```python
from build123d import *

# Parameters (mm, degrees)
P_IDAT_VYSUNUT_M1_DEPTH = 6
M6_D_RA_S_V_L_1_D       = 6.6
SKICA5_W                = 8
SKICA5_H                = 8
P_IDAT_VYSUNUT_M2_DEPTH = 2


with BuildPart() as part:
    # Skica1 → Přidat vysunutím1 (new body)
    with BuildSketch(Plane.XY):
        with BuildLine():
            Line((0, 0), (57, 0))
            ThreePointArc((57, 0), (59.121320344, 0.878679656), (60, 3))
            Line((60, 3), (60, 27))
            ThreePointArc((60, 27), (59.121320344, 29.121320344), (57, 30))
            Line((57, 30), (33, 30))
            ThreePointArc((33, 30), (30.878679656, 30.878679656), (30, 33))
            Line((30, 33), (30, 57))
            ThreePointArc((30, 57), (29.121320344, 59.121320344), (27, 60))
            Line((27, 60), (3, 60))
            ThreePointArc((3, 60), (0.878679656, 59.121320344), (0, 57))
            Line((0, 57), (0, 0))
        make_face()
    extrude(amount=P_IDAT_VYSUNUT_M1_DEPTH)

    # M6 díra s vůlí1 (through all)
    with Locations(Plane.XY.offset(6)):
        with Locations((45, 15), (15, 45)):
            Hole(M6_D_RA_S_V_L_1_D / 2)

    # Skica5 → Přidat vysunutím2 (add)
    with BuildSketch(Plane.XY.offset(6)):
        with BuildLine():
            ThreePointArc((19, 41.225082782), (15, 39.5), (11, 41.225082782))
            Line((11, 41.225082782), (11, 32.5))
            Line((11, 32.5), (19, 32.5))
            Line((19, 32.5), (19, 41.225082782))
        make_face()
        with BuildLine():
            Line((19, 57.5), (11, 57.5))
            Line((11, 57.5), (11, 48.774917218))
            ThreePointArc((11, 48.774917218), (15, 50.5), (19, 48.774917218))
            Line((19, 48.774917218), (19, 57.5))
        make_face()
        with BuildLine():
            Line((41.225082782, 19), (32.5, 19))
            Line((32.5, 19), (32.5, 11))
            Line((32.5, 11), (41.225082782, 11))
            ThreePointArc((41.225082782, 11), (39.5, 15), (41.225082782, 19))
        make_face()
        with BuildLine():
            Line((57.5, 19), (48.774917218, 19))
            ThreePointArc((48.774917218, 19), (50.050348735, 17.178067412), (50.5, 15))
            ThreePointArc((50.5, 15), (50.050348735, 12.821932588), (48.774917218, 11))
            Line((48.774917218, 11), (57.5, 11))
            Line((57.5, 11), (57.5, 19))
        make_face()
        with Locations((15, 15)):
            Rectangle(SKICA5_W, SKICA5_H)
    extrude(amount=P_IDAT_VYSUNUT_M2_DEPTH)


solid = part.part
```
The model under review builds one solid part; all positions refer to its coordinate system, in mm. A direction names the side the tool comes from. Round coordinates to 2 decimals unless told otherwise and drop trailing zeros. Write each loop counter-clockwise with the first axis right and the second up, starting at its lowest first coordinate (ties: lowest second). Pieces come first, ordered by that corner, then holes. Notation, with made-up numbers: (52, 78) -> (89, 78) arc R15 cw to (89, 90) -> close; hole circle Ø6 at (13.5, 78.25). An arc over 180 degrees is marked (long way). Use CSV: the item, a comma, the result in double quotes.
Q1. Consider section D-D (z = 3). Give the boundary of the cut face in (x, y).
Checks:
outline,"(0, 0) -> (57, 0) arc R3 ccw to (60, 3) -> (60, 27) arc R3 ccw to (57, 30) -> (33, 30) arc R3 cw to (30, 33) -> (30, 57) arc R3 ccw to (27, 60) -> (3, 60) arc R3 ccw to (0, 57) -> close; hole circle Ø6.6 at (15, 45); hole circle Ø6.6 at (45, 15)"
Q2. Consider section A-A (y = 45). Give the boundary of the cut face in (x, z), then the cut area to 3 significant figures.
Checks:
outline,"(0, 0) -> (11.7, 0) -> (11.7, 6) -> (0, 6) -> close; (18.3, 0) -> (30, 0) -> (30, 6) -> (18.3, 6) -> close"
area,"140 mm²"
Q3. For pin 1 Ø5 at (x, y) = (6, 6) entering from +Z; pin 2 Ø1 at (y, z) = (52, 7) entering from +X; pin 3 Ø1.8 at (x, z) = (41, 4) entering from +Y, all flat-tipped, find the tip position at first contact; note any pin that passes through.
Checks:
pin 1,"z = 6"
pin 2,"x = 19"
pin 3,"y = 30"
Q4. Consider section B-B (z = 6.75). Give the boundary of the cut face in (x, y), then the cut area to 3 significant figures.
Checks:
outline,"(11, 11) -> (19, 11) -> (19, 19) -> (11, 19) -> close; (11, 32.5) -> (19, 32.5) -> (19, 41.23) arc R5.5 cw to (11, 41.23) -> close; (11, 48.77) arc R5.5 cw to (19, 48.77) -> (19, 57.5) -> (11, 57.5) -> close; (32.5, 11) -> (41.23, 11) arc R5.5 cw to (41.23, 19) -> (32.5, 19) -> close; (48.77, 11) -> (57.5, 11) -> (57.5, 19) -> (48.77, 19) arc R5.5 cw to start"
area,"305 mm²"
Q5. Mouldability with a two-part tool opening along X and no side actions: class faces 1 (the cylindrical face through (59.14, 29.1, 2.96)), 2 (the flat face through (19, 15, 7)), 3 (the flat face through (53, 19, 7)) as released by +X, released by -X, zero draft, split by the parting line, or undercut.
Checks:
face 1,"released by +X"
face 2,"undercut"
face 3,"zero draft"
Q6. For faces 4 (the flat face through (19, 37, 7)), 5 (the flat face through (32.5, 15, 7)), 6 (the flat face through (30, 45, 3)), 7 (the cylindrical face through (39.5, 14.9, 7)), list the 3-axis set-ups (+Z, -Z, +X, -X, +Y, -Y) from which the entire face can be reached by the end or side of a thin tool; tool diameter is ignored.
Checks:
face 4,"+Z, +X, +Y, -Y"
face 5,"+Z, +Y, -Y"
face 6,"+Z, -Z, +X, +Y"
face 7,"+Z"
Q7. To check wall thickness, follow probe 1 along Y at (x, z) = (15, 2.75); probe 2 along Z at (x, y) = (25.5, 47); probe 3 along X at (y, z) = (35.5, 7). State the ranges of each line that lie inside material, in increasing order. Write a range as [from, to].
Checks:
probe 1,"[0, 41.7], [48.3, 60]"
probe 2,"[0, 6]"
probe 3,"[11, 19]"
Q8. Consider section C-C (x = 15). Give the boundary of the cut face in (y, z), then the cut area to 3 significant figures.
Checks:
outline,"(0, 0) -> (41.7, 0) -> (41.7, 6) -> (39.5, 6) -> (39.5, 8) -> (32.5, 8) -> (32.5, 6) -> (19, 6) -> (19, 8) -> (11, 8) -> (11, 6) -> (0, 6) -> close; (48.3, 0) -> (60, 0) -> (60, 6) -> (57.5, 6) -> (57.5, 8) -> (50.5, 8) -> (50.5, 6) -> (48.3, 6) -> close"
area,"364 mm²"
